Read the model definition and answer for the solid it produces. Units are mm, in the model's axes. A direction names the side the tool comes from. Coordinates: 2 decimals unless noted, no trailing zeros. Write each loop counter-clockwise with the first axis right and the second up, starting at its lowest first coordinate (ties: lowest second). Pieces come first, ordered by that corner, then holes.
1) Each of these flat-tipped pins is pushed along its axis until it touches: pin 1 Ø6 at (x, y) = (0.5, -5) entering from -Z (3 decimals); pin 2 Ø6.5 at (y, z) = (-9, 64.5) entering from +X; pin 3 Ø3 at (y, z) = (-8.5, 40) entering from +X. Where does it stop, or does it pass through?
2) The part is cut by section A-A (y = -8). Determine the outline of the cut face in (x, z) (3 decimals).
3) The part is cut by section C-C (z = 32.5). Determine the outline of the cut face in (x, y).
4) Which of the six approach directions +Z, -Z, +X, -X, +Y, -Y give full straight-line access (tool end or side, diameter ignored) to faces 4 (the face through (-10.206, -6, 67)), 5 (the face through (-6.958, -6.261, 37.817)), 6 (the face through (10.206, -6, 67))?
5) Find the intervals of material crossed by line 1 (Z direction, x = 0, y = -3.5) (3 decimals); line 2 (X direction, y = -5.75, z = 0.5); line 3 (X direction, y = -9.25, z = 26), in increasing order.
6) The part is cut by section B-B (x = 0). Determine the outline of the cut face in (y, z) (3 decimals), then the cut area to 3 significant figures.
7) The part is cut by section D-D (x = 15.5). Determine the outline of the cut face in (y, z), then the cut area to 3 significant figures.
8) Determine the mould class of faces 1 (the face through (-7, -12.7, 41)), 2 (the face through (14.034, -6.261, 32.445)), 3 (the face through (15.748, -6.261, 4.959)) for opening direction X: +X half, -X half, draft (parallel to the pull), parting line (faces both ways), or undercut.
from build123d import *

# Parameters (mm, degrees)
F0_R     = 16.51
F1_DEPTH = 12.7


# Not quite as in the source:
# - a feature names something its author has since deleted; it is built from what else it names


with BuildPart() as f1:
    # F0 (on Front) → F1 (new body)
    with BuildSketch(Plane.XZ):
        with BuildLine():
            ThreePointArc((17.7553829843, 4.8845265973), (14.8425769227, 10.9000062062), (9.9745940638, 15.4796543328))
            ThreePointArc((9.9745940638, 15.4796543328), (0, 18.415), (-9.9745940638, 15.4796543328))
            ThreePointArc((-9.9745940638, 15.4796543328), (-14.8425769227, 10.9000062062), (-17.7553829843, 4.8845265973))
            Line((-17.7553829843, 4.8845265973), (-18.415, 0))
            ThreePointArc((-18.415, 0), (0, -18.415), (18.415, 0))
            Line((18.415, 0), (17.7553829843, 4.8845265973))
        make_face()
        Circle(F0_R, mode=Mode.SUBTRACT)
        with BuildLine():
            ThreePointArc((-17.7553829843, 4.8845265973), (-14.8425769227, 10.9000062062), (-9.9745940638, 15.4796543328))
            Line((-9.9745940638, 15.4796543328), (-3.8560049814, 60.7883871295))
            Line((-3.8560049814, 60.7883871295), (-10.2060049814, 60.7883871295))
            Line((-10.2060049814, 60.7883871295), (-17.7553829843, 4.8845265973))
        make_face()
        with BuildLine():
            Line((3.8560049814, 60.7883871295), (9.9745940638, 15.4796543328))
            ThreePointArc((9.9745940638, 15.4796543328), (14.8425769227, 10.9000062062), (17.7553829843, 4.8845265973))
            Line((17.7553829843, 4.8845265973), (10.2060049814, 60.7883871295))
            Line((10.2060049814, 60.7883871295), (3.8560049814, 60.7883871295))
        make_face()
        with BuildLine():
            ThreePointArc((18.415, 0), (18.2493507098, 2.4644317137), (17.7553829843, 4.8845265973))
            Line((17.7553829843, 4.8845265973), (18.415, 0))
        make_face()
        with BuildLine():
            Line((-18.415, 0), (-17.7553829843, 4.8845265973))
            ThreePointArc((-17.7553829843, 4.8845265973), (-18.2493507098, 2.4644317137), (-18.415, 0))
        make_face()
        Polygon((0, 60.7883871295), (3.8560049814, 60.7883871295), (10.2060049814, 60.7883871295), (10.2060049814, 73.4883871295), (-10.2060049814, 73.4883871295), (-10.2060049814, 60.7883871295), (-3.8560049814, 60.7883871295), align=None)
    extrude(amount=F1_DEPTH)


solid = f1.part
Reported:
1. pin 1: stops at z = -18.415
1. pin 2: stops at x = 10.21
1. pin 3: stops at x = 13.22
2. outline: (-17.755, 4.885) arc R18.415 ccw (long way) to (17.755, 4.885) - (10.206, 60.788) - (10.206, 73.488) - (-10.206, 73.488) - (-10.206, 60.788) - close; hole circle Ø33.02 at (0, 0); hole (-9.975, 15.48) arc R18.415 cw to (9.975, 15.48) - (3.856, 60.788) - (-3.856, 60.788) - close
3. outline: (-14.03, -12.7) - (-7.68, -12.7) - (-7.68, 0) - (-14.03, 0) - close; (7.68, -12.7) - (14.03, -12.7) - (14.03, 0) - (7.68, 0) - close
4. face 4: +Z, -X, +Y, -Y
4. face 5: +Y, -Y
4. face 6: +Z, +X, +Y, -Y
5. line 1: z = -18.415 to -16.51, 16.51 to 18.415, 60.788 to 73.488
5. line 2: x = -18.41 to -16.5, 16.5 to 18.41
5. line 3: x = -14.9 to -8.55, 8.55 to 14.9
6. outline: (-12.7, -18.415) - (0, -18.415) - (0, -16.51) - (-12.7, -16.51) - close; (-12.7, 16.51) - (0, 16.51) - (0, 18.415) - (-12.7, 18.415) - close; (-12.7, 60.788) - (0, 60.788) - (0, 73.488) - (-12.7, 73.488) - close
6. area: 210 mm2
7. outline: (-12.7, -9.94) - (0, -9.94) - (0, -5.69) - (-12.7, -5.69) - close; (-12.7, 5.69) - (0, 5.69) - (0, 21.59) - (-12.7, 21.59) - close
7. area: 256 mm2
8. face 1: draft
8. face 2: +X half
8. face 3: undercut
